Verification items for this drawing (mm, ordinates from the low corner). A direction names the side the tool comes from. Round coordinates to 2 decimals unless told otherwise and drop trailing zeros. Loops run counter-clockwise (first coordinate to the right, second up) from the corner with the lowest first, then second, coordinate; pieces in that order, holes last. Notation, with made-up numbers: M 78,49.5 L 82,49.5 A29 ccw 82,69.5 Z; hole C -31.5,-22 d5. An arc over 180 degrees is marked long. Use one line per item in the form item = value. Start each with the question number.
1. Cross-section at B-B (x = 39). Record the boundary of the cut face in (y, z), then the cut area to 3 significant figures.
2. Cross-section at A-A (z = 8.97). Record the boundary of the cut face in (x, y), then the cut area to 3 significant figures.
3. Cross-section at C-C (z = 15.75). Record the boundary of the cut face in (x, y).
4. Go/stop test with flat-tipped pins: pin 1 (1 mm diameter, centred on x = 34.5, z = 2.5, fed in from +Y); pin 2 (3 mm diameter, centred on x = 46.5, y = 10, fed in from -Z). Record where each tip stops, or that it passes through.
5. Set-up check for the marked faces 1 and 2: record each of +Z, -Z, +X, -X, +Y, -Y from which the full face is reachable in a straight line by a thin tool's end or side.
6. Material ranges on line 1 (X direction, y = 0.9, z = 8.97); line 2 (Y direction, x = 47.5, z = 13.5); line 3 (Z direction, x = 36, y = 11.75), recorded low to high.
7. Cross-section at D-D (y = 7). Record the boundary of the cut face in (x, z), then the cut area to 3 significant figures.
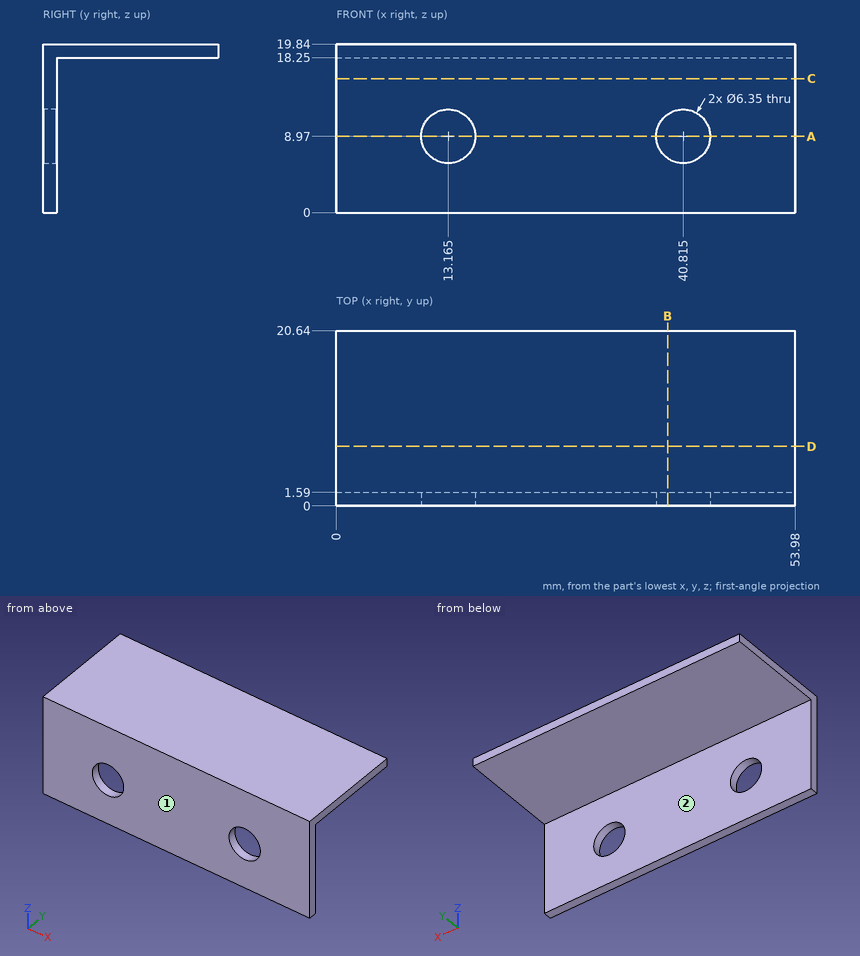
Reported:
q1.outline = M 0,0 L 1.59,0 L 1.59,6.36 L 0,6.36 Z; M 0,11.58 L 1.59,11.58 L 1.59,18.25 L 20.64,18.25 L 20.64,19.84 L 0,19.84 Z
q1.area = 53.6 mm²
q2.outline = M 0,0 L 9.99,0 L 9.99,1.59 L 0,1.59 Z; M 16.34,0 L 37.64,0 L 37.64,1.59 L 16.34,1.59 Z; M 43.99,0 L 53.98,0 L 53.98,1.59 L 43.99,1.59 Z
q2.area = 65.6 mm²
q3.outline = M 0,0 L 53.98,0 L 53.98,1.59 L 0,1.59 Z
q4.pin_1 = 1.59
q4.pin_2 = 18.25
q5.face_1 = +Z, -Z, +X, -X, -Y
q5.face_2 = -Z, +X, -X, +Y
q6.line_1 = 0 to 9.99, 16.34 to 37.64, 43.99 to 53.98
q6.line_2 = 0 to 1.59
q6.line_3 = 18.25 to 19.84
q7.outline = M 0,18.25 L 53.98,18.25 L 53.98,19.84 L 0,19.84 Z
q7.area = 85.8 mm²
